Input: dimensioned drawing with shaded views. Units: mm. Origin: part minimum x, y, z. A direction names the side the tool comes from. Coordinates: 2 decimals unless noted, no trailing zeros. Order: outer loops, then holes, each group sorted by start corner. A loop starts at its lowest first (then second) coordinate and runs counter-clockwise, first axis right, second up. Notation, with made-up numbers: M 83,42 L 104,42 A14 ccw 104,65 Z; hole C -30.75,87 d2. An arc over 180 degrees is marked long. Write item = value, one per line.
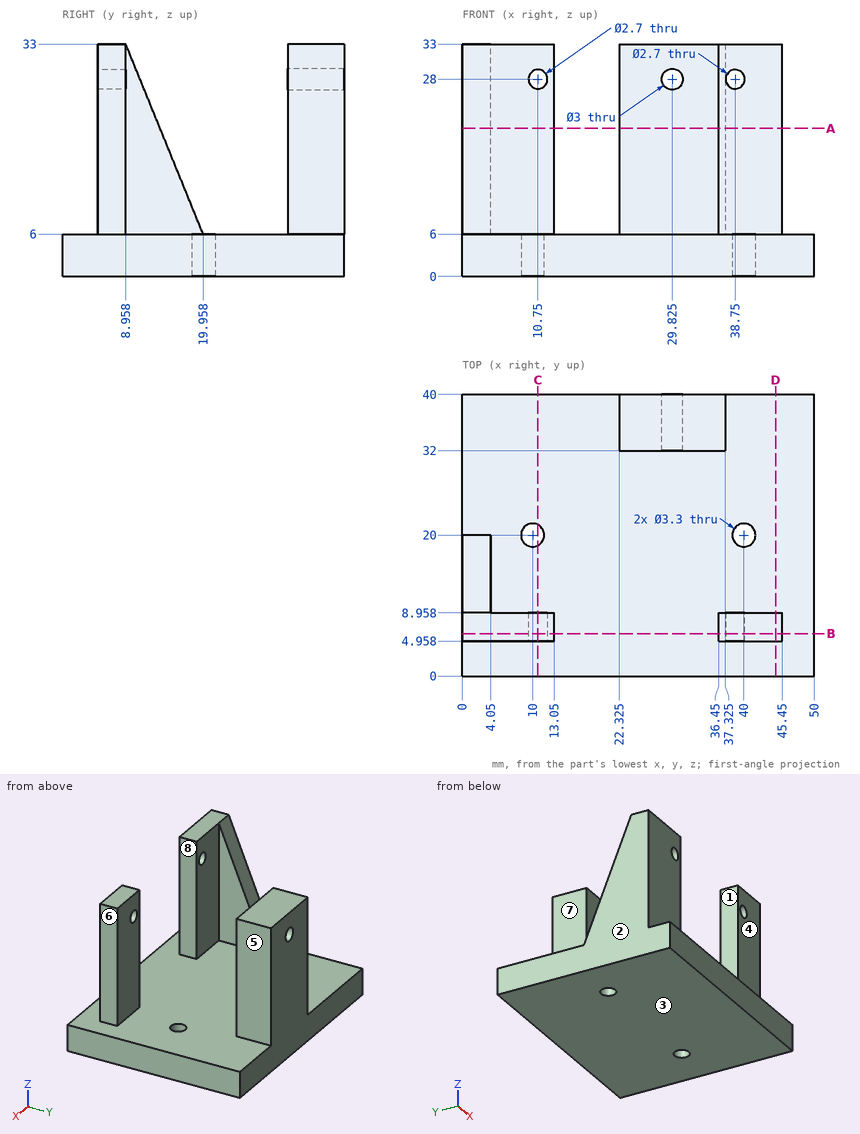
1) Pin query (flat end, axial travel): pin 1 (6 mm diameter, centred on x = 9, z = 18.5, fed in from -Y); pin 2 (2.5 mm diameter, centred on y = 37, z = 24.5, fed in from +X) (3 decimals); pin 3 (4.5 mm diameter, centred on y = 6.5, z = 21.5, fed in from +X). Return the tip coordinate at first contact, or that it passes through.
Numbers:
pin_1 = 4.96
pin_2 = 37.325
pin_3 = 45.45
2) Section B-B, the plane y = 6. Return loops of the section in (x, z), and give its area (3 significant figures).
Numbers:
outline = M 0,0 L 50,0 L 50,6 L 45.45,6 L 45.45,33 L 36.45,33 L 36.45,6 L 13.05,6 L 13.05,33 L 0,33 Z; hole C 10.75,28 d2.7; hole C 38.75,28 d2.7
area = 884 mm²
3) Line query: L1, parallel to Z at x = 10.75, y = 6.5; L2, parallel to Y at x = 10, z = 1.5; L3, parallel to X at y = 6, z = 12.5. Output: solid intervals per line, ascending.
Numbers:
L1 = 0 to 26.65, 29.35 to 33
L2 = 0 to 18.35, 21.65 to 40
L3 = 0 to 13.05, 36.45 to 45.45
4) Set-up query: the marked faces 4, 5, 6, 7 and 8. Return all of +Z, -Z, +X, -X, +Y, -Y with unobstructed straight access to the full face (end or side cutting, diameter ignored); none if empty.
Numbers:
face_4 = +Z, +X, -X, -Y
face_5 = +Z, +X, +Y
face_6 = +Z, +X, +Y, -Y
face_7 = +Z, -X, +Y, -Y
face_8 = +Z, +Y, -Y
5) Section D-D, the plane x = 44.5. Return loops of the section in (y, z).
Numbers:
outline = M 0,0 L 40,0 L 40,6 L 8.96,6 L 8.96,33 L 4.96,33 L 4.96,6 L 0,6 Z
6) Section A-A, the plane z = 21. Give the number of separate pieces and of enclosed holes in the cut face, and give its area (3 significant figures).
Numbers:
separate_pieces = 3
enclosed_holes = 0
area = 228 mm²
7) Mould query, pull axis X, two halves, no side actions, for the marked faces 1, 2 and 3. Classes: pulls with the +X half, pulls with the -X half, needs draft (parallel to the pull), parting line crosses it, or undercut.
Numbers:
face_1 = undercut
face_2 = pulls with the -X half
face_3 = needs draft
8) Section C-C, the plane x = 10.75. Return loops of the section in (y, z).
Numbers:
outline = M 0,0 L 18.53,0 L 18.53,6 L 8.96,6 L 8.96,26.65 L 4.96,26.65 L 4.96,6 L 0,6 Z; M 4.96,29.35 L 8.96,29.35 L 8.96,33 L 4.96,33 Z; M 21.47,0 L 40,0 L 40,6 L 21.47,6 Z
